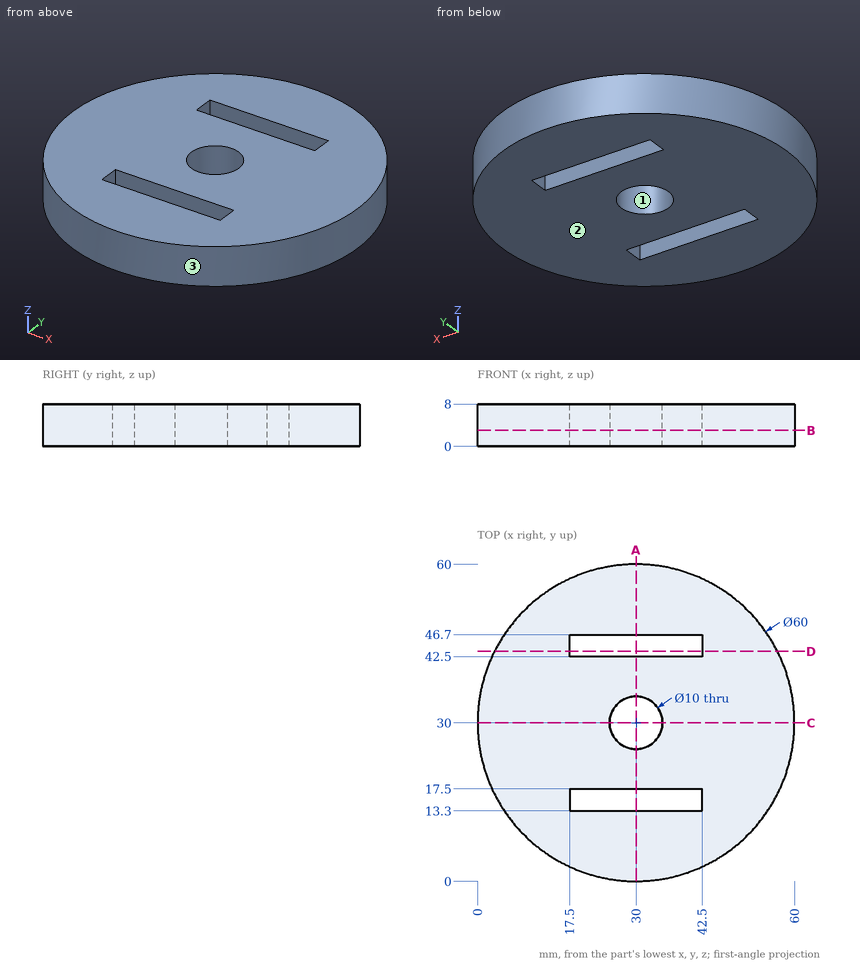
Geometry: see drawing. Coordinates: mm, zero at the bounding-box minimum. Give positions to 0.01 mm unless a question says otherwise; leave off trailing zeros. Order: outer loops, then holes, each group sorted by start corner. A loop starts at its lowest first (then second) coordinate and runs counter-clockwise, first axis right, second up. Notation, with made-up numbers: (-10, -21.5) - (40, -21.5) arc R24 cw to (40, -5.5) - close; hole circle Ø8 at (70.25, 87.25). An arc over 180 degrees is marked (long way). Use a Markdown table: item, result.
(1) Line query: line 1 (Y direction, x = 30, z = 3.5); line 2 (X direction, y = 30, z = 5.5); line 3 (Y direction, x = 40.5, z = 5.5). Output: solid intervals per line, ascending. Write a range as from..to.
Computed values:
| item | result |
|---|---|
| line 1 | y = 0..13.3, 17.5..25, 35..42.5, 46.7..60 |
| line 2 | x = 0..25, 35..60 |
| line 3 | y = 1.9..13.3, 17.5..42.5, 46.7..58.1 |
(2) Section query C-C (y = 30). Output: boundary loops of the cut face in (x, z), then the cut area to 3 significant figures.
Computed values:
| item | result |
|---|---|
| outline | (0, 0) - (25, 0) - (25, 8) - (0, 8) - close; (35, 0) - (60, 0) - (60, 8) - (35, 8) - close |
| area | 400 mm2 |
(3) Pin query (flat end, axial travel): pin 1 (2 mm diameter, centred on x = 34, z = 2, fed in from +Y); pin 2 (4.5 mm diameter, centred on y = 43.5, z = 5.5, fed in from +X); pin 3 (1.3 mm diameter, centred on y = 16, z = 4.5, fed in from -X). Return the tip coordinate at first contact, or that it passes through.
Computed values:
| item | result |
|---|---|
| pin 1 | stops at y = 59.85 |
| pin 2 | stops at x = 57.81 |
| pin 3 | stops at x = 3.13 |
(4) Draft query along Y for the marked faces 1, 2 and 3. Return one class per face: released by +Y, released by -Y, zero draft, split by the parting line, or undercut.
Computed values:
| item | result |
|---|---|
| face 1 | undercut |
| face 2 | zero draft |
| face 3 | split by the parting line |
(5) Section query B-B (z = 3). Output: boundary loops of the cut face in (x, y).
Computed values:
| item | result |
|---|---|
| outline | circle Ø60 at (30, 30); hole (17.5, 13.3) - (42.5, 13.3) - (42.5, 17.5) - (17.5, 17.5) - close; hole (17.5, 42.5) - (42.5, 42.5) - (42.5, 46.7) - (17.5, 46.7) - close; hole circle Ø10 at (30, 30) |
(6) Section query D-D (y = 43.5). Output: boundary loops of the cut face in (x, z).
Computed values:
| item | result |
|---|---|
| outline | (3.21, 0) - (17.5, 0) - (17.5, 8) - (3.21, 8) - close; (42.5, 0) - (56.79, 0) - (56.79, 8) - (42.5, 8) - close |
(7) Section query A-A (x = 30). Output: boundary loops of the cut face in (y, z).
Computed values:
| item | result |
|---|---|
| outline | (0, 0) - (13.3, 0) - (13.3, 8) - (0, 8) - close; (17.5, 0) - (25, 0) - (25, 8) - (17.5, 8) - close; (35, 0) - (42.5, 0) - (42.5, 8) - (35, 8) - close; (46.7, 0) - (60, 0) - (60, 8) - (46.7, 8) - close |
